from build123d import *

# Parameters (mm, degrees)
BOSS_EXTRUDE1_DEPTH      = 107
SKETCH7_W                = 87
SKETCH7_H                = 20
CUT_EXTRUDE4_DEPTH       = 25
SKETCH8_R                = 5
SKETCH8_R_2              = 3
BOSS_EXTRUDE3_DEPTH      = 25
BOSS_EXTRUDE4_DEPTH      = 3
BOSS_EXTRUDE4_DEPTH_BACK = 3
BOSS_EXTRUDE4_START      = 11.5


with BuildPart() as part:
    # Sketch2 → Boss-Extrude1 (new body)
    with BuildSketch(Plane(origin=(0, 0, 0), x_dir=(0, 0, -1), z_dir=(1, 0, 0))):
        Polygon((0, 0), (-23, 0), (-23, -23), (-20, -23), (-20, -3), (0, -3), align=None)
    extrude(amount=-BOSS_EXTRUDE1_DEPTH)

    # Sketch7 → Cut-Extrude4 (cut)
    with BuildSketch(Plane.XY.offset(23)):
        with Locations((-63.5, -13)):
            Rectangle(SKETCH7_W, SKETCH7_H)
    extrude(amount=-CUT_EXTRUDE4_DEPTH, mode=Mode.SUBTRACT)

    # Sketch8 → Boss-Extrude3 (add)
    with BuildSketch(Plane.XY.offset(23)):
        with Locations((-10, -13)):
            Circle(SKETCH8_R)
        with Locations(Location((-10, -13, 0), (0, 0, 270))):
            Circle(SKETCH8_R_2, mode=Mode.SUBTRACT)
    extrude(amount=BOSS_EXTRUDE3_DEPTH)

    # Sketch9 → Boss-Extrude4 (add, two sides: drawn at the far end of the back side and taken through both)
    with BuildSketch(Plane.XY.offset(BOSS_EXTRUDE4_START - BOSS_EXTRUDE4_DEPTH_BACK)):
        Polygon((-107, 0), (-107, 1), (-110.55, 1), (-110.55, 0), (-113.55, 0), (-113.55, 1.75), (-110.55, 1.75), (-106, 1.75), (-106, 0), align=None)
    extrude(amount=BOSS_EXTRUDE4_DEPTH + BOSS_EXTRUDE4_DEPTH_BACK)


solid = part.part
Read the model definition and answer for the solid it produces. Units are mm, in the model's axes. A direction names the side the tool comes from. Give positions to 0.01 mm unless a question says otherwise; leave off trailing zeros. Loops run counter-clockwise (first coordinate to the right, second up) from the corner with the lowest first, then second, coordinate; pieces in that order, holes last. Notation, with made-up numbers: M 56,-32.75 L 101,-32.75 A24 cw 101,-12.75 Z; hole C -33,-20 d3. An arc over 180 degrees is marked long. Write each question's results on one line, items separated by ' | '.
1. Section A-A on x = -10 is taken. Give the vertices of the cut face in (y, z).
Values:
outline: M -23,20 L -3,20 L -3,0 L 0,0 L 0,23 L -8,23 L -8,48 L -10,48 L -10,23 L -16,23 L -16,48 L -18,48 L -18,23 L -23,23 Z
2. Section B-B on y = -13 is taken. Give the vertices of the cut face in (x, z).
Values:
outline: M -20,20 L 0,20 L 0,23 L -5,23 L -5,48 L -7,48 L -7,23 L -13,23 L -13,48 L -15,48 L -15,23 L -20,23 Z
3. Section C-C on z = 39.5 is taken. Give the vertices of the cut face in (x, y).
Values:
outline: C -10,-13 d10; hole C -10,-13 d6
4. The mould has two halves that part along X. Classify faces 6 (the face through (-5.23, -11.5, 35.33)), 7 (the face through (-10, -13, 20)), 8 (the face through (-10, -10, 35)): pulls with the +X half, pulls with the -X half, needs draft (parallel to the pull), parting line crosses it, or undercut.
Values:
face 6: parting line crosses it | face 7: needs draft | face 8: undercut
5. A tool of negligible diameter and unlimited length cuts with its end or side. For faces 1 (the face through (-10, -13, 23)), 2 (the face through (-10, -23, 22)), 3 (the face through (-109, 1, 11)), 4 (the face through (-110, 1.75, 11)), 5 (the face through (-112, 0, 11)), from which of +Z, -Z, +X, -X, +Y, -Y can it reach the whole face along a straight path? Write none if from no direction.
Values:
face 1: +Z | face 2: +Z, -Z, +X, -X, -Y | face 3: +Z, -Z, -Y | face 4: +Z, -Z, +X, -X, +Y | face 5: +Z, -Z, -X, -Y
6. Section D-D on z = 4 is taken. Give the vertices of the cut face in (x, y).
Values:
outline: M -107,-3 L 0,-3 L 0,0 L -107,0 Z
7. Straight lines are drawn through the part: line 1 (Z direction, x = -60, y = -1.5); line 2 (X direction, y = -18.75, z = 22.5); line 3 (Y direction, x = -66, z = 20.5). For each, find the intervals that lie inside material, in ascending order. Write a range as [from, to].
Values:
line 1: z = [0, 23] | line 2: x = [-20, 0] | line 3: y = [-3, 0]
8. Given pin 1 (11.5 mm diameter, centred on x = -66, z = 8, fed in from -Y); pin 2 (12 mm diameter, centred on x = -88.5, z = 28, fed in from +Y); pin 3 (1.8 mm diameter, centred on x = -9, y = -14.5, fed in from +Z); pin 4 (4.5 mm diameter, centred on y = -1.5, z = 11, fed in from -X), each flat-ended and moving along its own axis, determine where each tip first touches the part or whether it passes through.
Values:
pin 1: stops at y = -3 | pin 2: stops at y = 0 | pin 3: stops at z = 23 | pin 4: stops at x = -113.55
